```python
from build123d import *

# Parameters (mm, degrees)
F0_R     = 8.4
F0_R_2   = 3.4
F1_DEPTH = 12.5
F4_R     = 8.25
F4_R_2   = 3.25
F8_D     = 2.5
F8_DEPTH = 101
F8_TIP   = 0.7510757738


with BuildPart() as f1:
    # F0 (on Front) → F1 (new body, symmetric)
    with BuildSketch(Plane.XZ):
        Circle(F0_R)
        Circle(F0_R_2, mode=Mode.SUBTRACT)
    extrude(amount=F1_DEPTH, both=True)

    # F4 (on face) → F5 (join, up to the next surface of F1)
    with BuildSketch(Plane(origin=(-21.7175651559, 9.2185594781, 0), x_dir=(-0.3907311285, -0.9205048535, 0), z_dir=(-0.9205048535, 0.3907311285, 0))):
        with Locations((3.2821414793, 0)):
            Circle(F4_R)
        with Locations((3.2821414793, 0)):
            Circle(F4_R_2, mode=Mode.SUBTRACT)
    extrude(until=Until.NEXT, dir=(0.9205048535, -0.3907311285, 0))

    # F6: F1 across plane


with BuildPart() as f1_1:
    add(f1.part)
    add(f1.part.mirror(Plane.YZ))

    # F8 (one way)
    with BuildSketch(Plane(origin=(0, 0, 0), x_dir=(1, 0, 0), z_dir=(0, 0, -1))):
        with Locations((0, -2.8046087828)):
            Circle(F8_D / 2)
    extrude(amount=-F8_DEPTH, mode=Mode.SUBTRACT)
    with Locations(Plane(origin=(0, 0, 0), x_dir=(1, 0, 0), z_dir=(0, 0, -1))):
        with Locations((0, -2.8046087828)):
            with Locations((0, 0, -(F8_DEPTH + F8_TIP / 2))):  # 118° drill point
                Cone(0, F8_D / 2, F8_TIP, mode=Mode.SUBTRACT)


solid = f1_1.part
```
Design review of the part built by this model. Coordinates are the model's own, in mm. A direction names the side the tool comes from. Coordinates: 2 decimals unless noted, no trailing zeros. Write each loop counter-clockwise with the first axis right and the second up, starting at its lowest first coordinate (ties: lowest second). Pieces come first, ordered by that corner, then holes. Notation, with made-up numbers: M 80,22 L 104,22 A25 cw 104,45 Z; hole C -8,30.25 d10. An arc over 180 degrees is marked long. Answer as a JSON object with one key per item and string values.
Item 1: Draft analysis for pull direction X (two halves, no side actions). For faces 1 (the flat face through (24.4, 2.9, 0.1)), 2 (the cylindrical face through (-16.387, 0.023, 0.976)), 3 (the cylindrical face through (16.387, 0.023, 0.976)), 4 (the flat face through (-24.4, 2.9, 0.1)), state which applies: pulls with the +X half, pulls with the -X half, needs draft (parallel to the pull), parting line crosses it, or undercut.
Outcome:
{"face 1": "pulls with the +X half", "face 2": "undercut", "face 3": "undercut", "face 4": "pulls with the -X half"}
Item 2: Add section D-D, the plane y = 11.75. State how many separate pieces and enclosed holes the cut face has, and give its area (3 significant figures).
Outcome:
{"separate pieces": "3", "enclosed holes": "1", "area": "273 mm²"}
Item 3: Insertion check: pin 1 Ø2 at (x, y) = (0, 2.8) entering from +Z; pin 2 Ø8 at (x, z) = (0, 0) entering from +Y; pin 3 Ø6 at (x, z) = (-14, 4) entering from +Y; pin 4 Ø10 at (x, y) = (3, 4) entering from -Z. Each pin has a flat end and moves straight along its axis. Give the tip position at first contact, or say it passes through.
Outcome:
{"pin 1": "z = -3.25", "pin 2": "y = 12.5", "pin 3": "y = 12.03", "pin 4": "z = -8.4"}
Item 4: Wall thickness on probe 1 along Y at (x, z) = (0, 6.5); probe 2 along X at (y, z) = (7, 4.75); probe 3 along X at (y, z) = (-1.75, 1.75): over which ranges is each line inside the solid? List them lowest first.
Outcome:
{"probe 1": "-12.5 to 1.55, 4.05 to 12.5", "probe 2": "-22.66 to -7.63, -6.93 to 6.93, 7.63 to 22.66", "probe 3": "-24.91 to -11.29, -8.22 to -2.92, 2.92 to 8.22, 11.29 to 24.91"}
Item 5: Add section B-B, the plane z = -1.25. Give the boundary of the cut face in (x, y), and give its area (3 significant figures).
Outcome:
{"outline": "M -26.19,-1.31 L -8.31,-8.9 L -8.31,-12.5 L -3.16,-12.5 L -3.16,12.5 L -8.31,12.5 L -8.31,8.82 L -19.81,13.7 L -21.83,8.96 L -8.31,3.22 L -8.31,-3.3 L -24.17,3.44 Z; M 3.16,-12.5 L 8.31,-12.5 L 8.31,-8.9 L 26.19,-1.31 L 24.17,3.44 L 8.31,-3.3 L 8.31,3.22 L 21.83,8.96 L 19.81,13.7 L 8.31,8.82 L 8.31,12.5 L 3.16,12.5 Z", "area": "586 mm²"}
Item 6: Add section C-C, the plane z = 6.25. Give the boundary of the cut face in (x, y), and give its area (3 significant figures).
Outcome:
{"outline": "M -25.1,1.24 L -5.61,-7.03 L -5.61,-12.5 L 5.61,-12.5 L 5.61,-7.03 L 25.1,1.24 L 20.9,11.15 L 5.61,4.67 L 5.61,12.5 L -5.61,12.5 L -5.61,4.67 L -20.9,11.15 Z; hole C 0,2.8 d2.5", "area": "683 mm²"}
Item 7: Machinability: for faces 5 (the cylindrical face through (-0.163, 1.565, 5.746)), 6 (the flat face through (4, 12.5, 0)), 7 (the cylindrical face through (8.4, 0, 0)), which of the approach directions +Z, -Z, +X, -X, +Y, -Y give a long, thin tool a straight path to every point of the face, cutting with its end or side? Answer none if there is none.
Outcome:
{"face 5": "+Z", "face 6": "+Z, -Z, +Y", "face 7": "none"}
Item 8: Add section A-A, the plane x = 0. Give the boundary of the cut face in (y, z), and give its area (4 significant figures).
Outcome:
{"outline": "M -12.5,-8.4 L 12.5,-8.4 L 12.5,-3.4 L -12.5,-3.4 Z; M -12.5,3.4 L 1.55,3.4 L 1.55,8.4 L -12.5,8.4 Z; M 4.05,3.4 L 12.5,3.4 L 12.5,8.4 L 4.05,8.4 Z", "area": "237.5 mm²"}
